Geometry check sheet. Reference: the model listing, model coordinates, mm. A direction names the side the tool comes from. Coordinates: 2 decimals unless noted, no trailing zeros. Order: outer loops, then holes, each group sorted by start corner. A loop starts at its lowest first (then second) coordinate and runs counter-clockwise, first axis right, second up. Notation, with made-up numbers: (-30, -19.75) - (-13, -19.75) arc R10 cw to (-13, -5.75) - close; hole circle Ø11 at (-28.5, 63.5). An arc over 180 degrees is marked (long way). Return JSON: item names as keys, results as strings. Group by question number.
Item 1: Section check D-D on x = -0.7. Enter the section's corners in (y, z) (3 decimals).
Item 2: Draft check along Z on faces 4 (the cylindrical face through (-0.35, 32.06, 3.62)), 5 (the cylindrical face through (-4.375, 18.565, 2.465)), 6 (the flat face through (4, 16, 0)). Enter one of: pulls with the +Z half, pulls with the -Z half, needs draft (parallel to the pull), parting line crosses it, or undercut.
Item 3: Section check C-C on z = 2.5. Enter the section's corners in (x, y) (3 decimals), then the cut area to 3 significant figures.
Item 4: Section check A-A on y = 0. Enter the section's corners in (x, z), then the cut area to 3 significant figures.
Item 5: Gauge pin test, flat ends, axial feed: pin 1 (2.5 mm diameter, centred on y = 29, z = 3, fed in from -X); pin 2 (1.9 mm diameter, centred on x = 13.8, z = 2.5, fed in from +Y); pin 3 (1 mm diameter, centred on y = 30.5, z = 2, fed in from +X). Record the tip position at first contact, or that the pin passes through.
Item 6: Scan lines: probe 1 along Y at (x, z) = (12.7, 2.3); probe 2 along X at (y, z) = (30.5, 3.25); probe 3 along X at (y, z) = (31, 2.5) (3 decimals). Record each from-to range of solid material in increasing order.
Item 7: Section check B-B on x = 13.8. Enter the section's corners in (y, z) (3 decimals), then the cut area to 3 significant figures.
Item 8: Tool access check on faces 1 (the flat face through (19, 1, 2)), 2 (the flat face through (-1, 28, 2)), 3 (the flat face through (-4.2, 28, 3)). Record the directions out of +Z, -Z, +X, -X, +Y, -Y that give a thin tool (end or side, any length) a straight path to the whole face; none if there is none.
from build123d import *

# Parameters (mm, degrees)
SKETCH1_W           = 38
SKETCH1_H           = 10
BOSS_EXTRUDE1_DEPTH = 5
SKETCH2_R           = 2.75
CUT_EXTRUDE1_DEPTH  = 5
SKETCH3_W           = 21.5
SKETCH3_H           = 31
BOSS_EXTRUDE2_DEPTH = 5
BOSS_EXTRUDE6_DEPTH = 5
SKETCH10_R          = 1.175
CUT_EXTRUDE4_DEPTH  = 8
FILLET2_R           = 2
BOSS_EXTRUDE7_DEPTH = 5


with BuildPart() as part:
    # Sketch1 → Boss-Extrude1 (new body)
    with BuildSketch(Plane.XY):
        Rectangle(SKETCH1_W, SKETCH1_H)
    extrude(amount=BOSS_EXTRUDE1_DEPTH)

    # Sketch2 → Cut-Extrude1 (cut)
    with BuildSketch(Plane.XY.offset(5)):
        with Locations((-12.7, 0)):
            Circle(SKETCH2_R)
        with Locations((12.7, 0)):
            Circle(SKETCH2_R)
    extrude(amount=-CUT_EXTRUDE1_DEPTH, mode=Mode.SUBTRACT)

    # Sketch3 → Boss-Extrude2 (add)
    with BuildSketch(Plane.XY.offset(5)):
        with Locations((6.55, 20.5)):
            Rectangle(SKETCH3_W, SKETCH3_H)
    extrude(amount=-BOSS_EXTRUDE2_DEPTH)

    # Sketch8 → Boss-Extrude6 (add)
    with BuildSketch(Plane.XY.offset(5)):
        Polygon((-4.2, 5), (-19, 5), (-4.2, 18.5), align=None)
    extrude(amount=-BOSS_EXTRUDE6_DEPTH)

    # Sketch10 → Cut-Extrude4 (cut)
    with BuildSketch(Plane(origin=(0, 36, 0), x_dir=(1, 0, 0), z_dir=(0, 1, 0))):
        with Locations(Location((-0.7, -2.5, 0), (0, 0, 270))):
            Circle(SKETCH10_R)
        with Locations(Location((13.8, -2.5, 0), (0, 0, 270))):
            Circle(SKETCH10_R)
    extrude(amount=-CUT_EXTRUDE4_DEPTH, mode=Mode.SUBTRACT)

    # Fillet2
    fillet2_edges = [part.edges().sort_by_distance(p)[0] for p in [
        (-4.2, 18.5, 2.5),
        (19, -5, 2.5),
        (-19, -5, 2.5),
        (-19, 5, 2.5),
    ]]
    fillet(fillet2_edges, radius=FILLET2_R)

    # Sketch11 → Boss-Extrude7 (add)
    with BuildSketch(Plane.XY.offset(5)):
        Polygon((19, 5), (17.3, 36), (17.3, 5), align=None)
    extrude(amount=-BOSS_EXTRUDE7_DEPTH)


solid = part.part
Computed:
{
 "1": {"outline": "(-5, 0) - (36, 0) - (36, 1.325) - (28, 1.325) - (28, 3.675) - (36, 3.675) - (36, 5) - (-5, 5) - close"},
 "2": {"face 4": "undercut", "face 5": "needs draft", "face 6": "pulls with the -Z half"},
 "3": {"outline": "(-19, -3) arc R2 ccw to (-17, -5) - (17, -5) arc R2 ccw to (19, -3) - (19, 5) - (17.3, 36) - (14.975, 36) - (14.975, 28) - (12.625, 28) - (12.625, 36) - (0.475, 36) - (0.475, 28) - (-1.875, 28) - (-1.875, 36) - (-4.2, 36) - (-4.2, 19.383) arc R2 cw to (-4.852, 17.905) - (-18.348, 5.595) arc R2 ccw to (-19, 4.117) - close; hole circle Ø5.5 at (-12.7, 0); hole circle Ø5.5 at (12.7, 0)", "area": "1,090 mm²"},
 "4": {"outline": "(-19, 0) - (-15.45, 0) - (-15.45, 5) - (-19, 5) - close; (-9.95, 0) - (9.95, 0) - (9.95, 5) - (-9.95, 5) - close; (15.45, 0) - (19, 0) - (19, 5) - (15.45, 5) - close", "area": "135 mm²"},
 "5": {"pin 1": "stops at x = -4.2", "pin 2": "stops at y = 28", "pin 3": "stops at x = 17.63"},
 "6": {"probe 1": "y = -5 to -2.75, 2.75 to 28", "probe 2": "x = -4.2 to -1.6, 0.2 to 12.9, 14.7 to 17.6", "probe 3": "x = -4.2 to -1.875, 0.475 to 12.625, 14.975 to 17.574"},
 "7": {"outline": "(-5, 0) - (-2.52, 0) - (-2.52, 5) - (-5, 5) - close; (2.52, 0) - (36, 0) - (36, 1.325) - (28, 1.325) - (28, 3.675) - (36, 3.675) - (36, 5) - (2.52, 5) - close", "area": "161 mm²"},
 "8": {"face 1": "+Z, -Z, +X, +Y, -Y", "face 2": "+Y", "face 3": "+Z, -Z, -X, +Y"}
}
